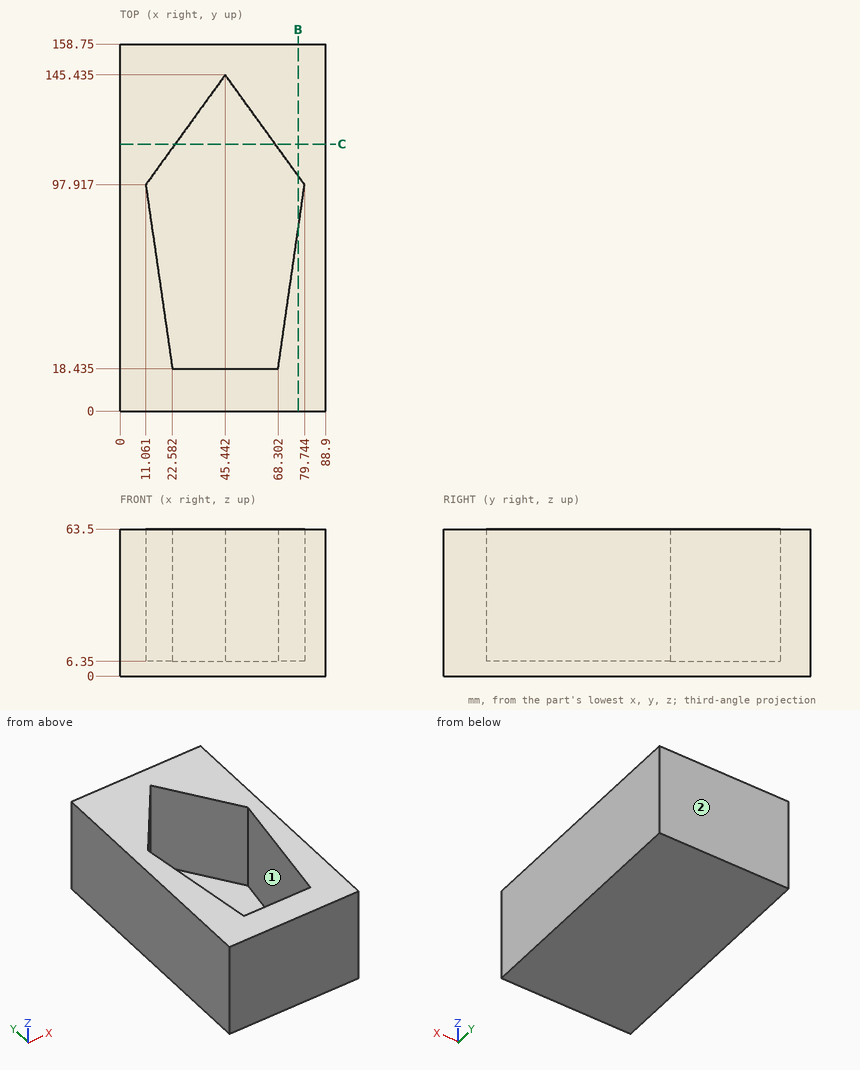
Drawing for the job (mm, zero at the part's lowest x, y, z). A direction names the side the tool comes from. Round coordinates to 2 decimals unless told otherwise and drop trailing zeros. Write each loop counter-clockwise with the first axis right and the second up, starting at its lowest first coordinate (ties: lowest second). Pieces come first, ordered by that corner, then holes. Notation, with made-up numbers: (-12, -32.75) - (20, -32.75) arc R19 ccw to (20, -5.75) - close; hole circle Ø2 at (34, -31.5). An arc over 180 degrees is marked (long way). Return JSON: item names as keys, results as strings. Group by question number.
Item 1: Flat gauge pin, fed straight in: pin 1 Ø3 at (x, y) = (44.5, 129) entering from +Z. Where does the tip first touch, or does it go through?
Item 2: Band-saw the part on B-B on x = 77. List the corners of the cut face in (y, z).
Item 3: Probe probe 1 along X at (y, z) = (131.5, 24); probe 2 along X at (y, z) = (33.5, 50); probe 3 along Z at (x, y) = (36.5, 77.5). List the from-to ranges inside material, lowest first.
Item 4: 3-axis set-ups, long thin cutter, end or side, ignore diameter. For the marked faces 1 and 2: which of +Z, -Z, +X, -X, +Y, -Y reach the whole face in a straight line?
Item 5: Band-saw the part on C-C on y = 115.5. List the corners of the cut face in (x, z), plus the area to 3 significant figures.
Resolved:
{
 "1": {"pin 1": "stops at z = 6.35"},
 "2": {"outline": "(0, 0) - (158.75, 0) - (158.75, 63.5) - (101.72, 63.5) - (101.72, 6.35) - (78.85, 6.35) - (78.85, 63.5) - (0, 63.5) - close"},
 "3": {"probe 1": "x = 0 to 35.36, 55.5 to 88.9", "probe 2": "x = 0 to 20.4, 70.47 to 88.9", "probe 3": "z = 0 to 6.35"},
 "4": {"face 1": "+Z", "face 2": "+Z, -Z, +X, -X, +Y"},
 "5": {"outline": "(0, 0) - (88.9, 0) - (88.9, 63.5) - (67.05, 63.5) - (67.05, 6.35) - (23.78, 6.35) - (23.78, 63.5) - (0, 63.5) - close", "area": "3,170 mm²"}
}
